Can you work these out from the drawing? Everything is in mm from the part's minimum corner. A direction names the side the tool comes from. Round coordinates to 2 decimals unless told otherwise and drop trailing zeros. Write each loop counter-clockwise with the first axis right and the second up, starting at its lowest first coordinate (ties: lowest second). Pieces come first, ordered by that corner, then holes.
Q1. If we section it at C-C (x = 16): Please give me the cut outline in (y, z).
Q2. For the marked faces 5 and 6, which set-ups out of +Z, -Z, +X, -X, +Y, -Y let a thin tool reach every point of the face, with its end or its side?
Q3. Please list where these lines run through material, in increasing order: line 1 along X through (y, z) = (3.75, 3.5); line 2 along Z through (x, y) = (22, 2).
Q4. If we section it at A-A (z = 20.5): Please give me the cut outline in (x, y).
Q5. If we section it at B-B (y = 2): Please give me the cut outline in (x, z).
Q6. We'd pull the mould along X, two halves only. Please class the marked faces 1, 2, 3 and 4: +X half, -X half, draft (parallel to the pull), parting line (faces both ways), or undercut.
Q7. I'm going to push a flat-ended pin straight in: pin 1 Ø2 at (x, y) = (36, 11) entering from -Z. Where does the tip first touch, or does it pass through?
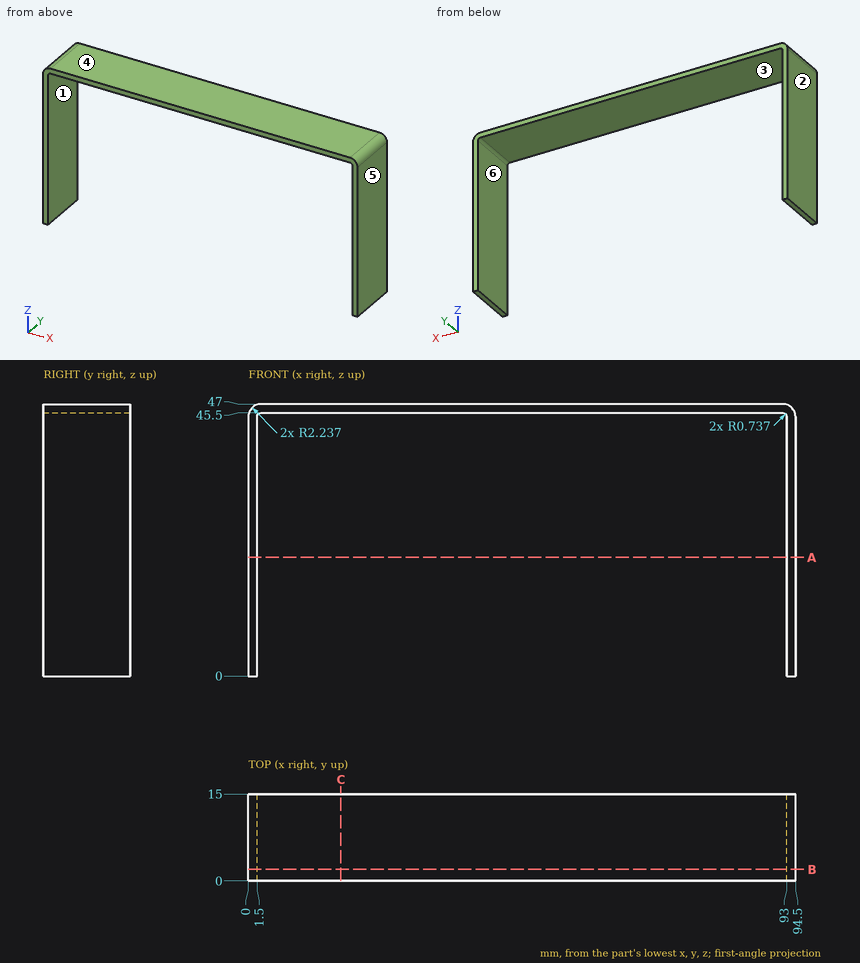
A:
1. outline: (0, 45.5) - (15, 45.5) - (15, 47) - (0, 47) - close
2. face 5: +Z, -Z, +X, +Y, -Y
2. face 6: -Z, +Y, -Y
3. line 1: x = 0 to 1.5, 93 to 94.5
3. line 2: z = 45.5 to 47
4. outline: (0, 0) - (1.5, 0) - (1.5, 15) - (0, 15) - close; (93, 0) - (94.5, 0) - (94.5, 15) - (93, 15) - close
5. outline: (0, 0) - (1.5, 0) - (1.5, 44.76) arc R0.74 cw to (2.24, 45.5) - (92.26, 45.5) arc R0.74 cw to (93, 44.76) - (93, 0) - (94.5, 0) - (94.5, 44.76) arc R2.24 ccw to (92.26, 47) - (2.24, 47) arc R2.24 ccw to (0, 44.76) - close
6. face 1: undercut
6. face 2: -X half
6. face 3: undercut
6. face 4: draft
7. pin 1: stops at z = 45.5
